Autodesk Inventor part; units mm, degrees
ref_plane "YZ Plane" through (0, 0, 0) normal (1, 0, 0) x (0, 1, 0)
ref_plane "XZ Plane" through (0, 0, 0) normal (0, 1, 0) x (-1, 0, 0)
ref_plane "XY Plane" through (0, 0, 0) normal (0, 0, 1) x (1, 0, 0)
sketch "Sketch1" plane through (0, 0, 0) normal (0, 1, 0) x (-1, 0, 0)
  line L0 (0, 0) -> (0, -152.4)
  line L1 (0, -152.4) -> (203.2, -152.4)
  line L2 (203.2, -152.4) -> (203.2, -31.75)
  line L3 (203.2, -31.75) -> (127, 0)
  line L4 (127, 0) -> (0, 0)
  dimension "d0" = 120.65
  dimension "d1" = 203.2
  dimension "d2" = 127
  dimension "d3" = 152.4
extrude "Extrusion1" add sketch "Sketch1" along normal blind 6.35
sketch "Sketch3" plane through (0, 6.35, 0) normal (0, 1, 0) x (1, 0, 0)
  line L0 (0, 0) -> (0, 152.4)
  line L1 (0, 152.4) -> (-203.2, 152.4)
  line L2 (-203.2, 152.4) -> (-203.2, 31.75)
  line L3 (-203.2, 31.75) -> (-127, 0)
  line L4 (-127, 0) -> (0, 0)
  line L5 (-19.05, 19.05) -> (-19.05, 133.35)
  line L6 (-19.05, 133.35) -> (-184.15, 133.35)
  line L7 (-184.15, 133.35) -> (-184.15, 50.8)
  line L8 (-19.05, 19.05) -> (-107.95, 19.05)
  line L9 (-107.95, 19.05) -> (-184.15, 50.8)
  circle A0 centre (-9.271, 15.875) radius 1.524
  circle A1 centre (-9.271, 136.525) radius 1.524
  circle A2 centre (-25.4, 143.129) radius 1.524
  circle A3 centre (-190.5, 143.129) radius 1.524
  circle A4 centre (-193.929, 47.625) radius 1.524
  circle A5 centre (-193.929, 136.525) radius 1.524
  circle A6 centre (-15.875, 9.271) radius 1.524
  circle A7 centre (-111.125, 9.271) radius 1.524
  dimension "d10" = 120.65
  dimension "d11" = 82.55
  dimension "d12" = 203.2
  dimension "d13" = 165.1
  dimension "d14" = 114.3
  dimension "d15" = 88.9
  dimension "d16" = 19.05
  dimension "d17" = 19.05
  dimension "d18" = 3.048
  dimension "d19" = 3.048
  dimension "d20" = 120.65
  dimension "d21" = 3.048
  dimension "d22" = 3.048
  dimension "d23" = 15.875
  dimension "d24" = 9.271
  dimension "d25" = 9.271
  dimension "d26" = 9.271
  dimension "d27" = 25.4
  dimension "d28" = 12.7
  dimension "d29" = 9.271
  dimension "d30" = 3.048
  dimension "d31" = 3.048
  dimension "d32" = 88.9
  dimension "d33" = 15.875
  dimension "d34" = 9.271
  dimension "d35" = 9.271
  dimension "d36" = 3.048
  dimension "d37" = 9.271
  dimension "d38" = 15.875
  dimension "d39" = 3.048
  dimension "d40" = 15.875
  dimension "d41" = 9.271
extrude "Extrusion2" cut sketch "Sketch3" against normal blind 6.35 contours L8 L9 L7 L6 L5 | A0 | A1 | A2 | A3 | A4 | A5 | A6 | A7
sketch "Sketch4" plane through (0, 6.35, 0) normal (0, 1, 0) x (1, 0, 0)
  circle A0 centre (-13.97, 44.45) radius 1.524
  circle A1 centre (-13.97, 107.95) radius 1.524
  circle A2 centre (-189.23, 92.075) radius 1.524
  line L0 (-107.95, 19.05) -> (-184.15, 50.8)
  line L1 (-184.15, 50.8) -> (-184.15, 133.35)
  line L2 (-19.05, 133.35) -> (-19.05, 19.05)
  point P0 (0, 0)
  dimension "d44" = 3.048
  dimension "d45" = 3.048
  dimension "d46" = 3.048
  dimension "d47" = 82.55
  dimension "d48" = 41.275
  dimension "d49" = 5.08
  dimension "d50" = 25.4
  dimension "d51" = 25.4
  dimension "d52" = 5.08
  dimension "d53" = 5.08
extrude "Extrusion3" cut sketch "Sketch4" against normal blind 6.35
properties part number "Panel"
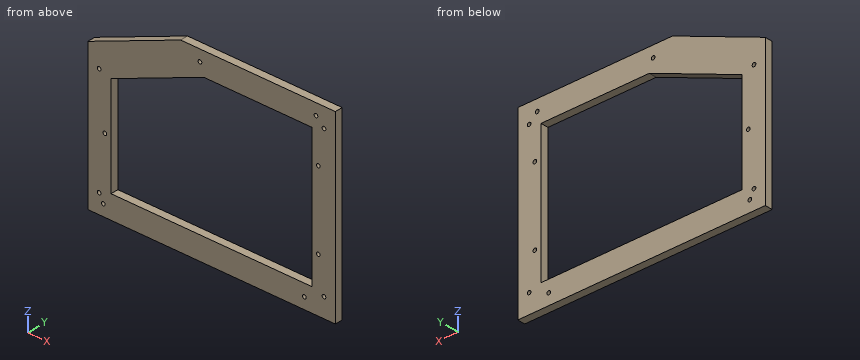
Design review of the part built by this model. Coordinates are the model's own, in mm. Give positions to 0.01 mm unless a question says otherwise; leave off trailing zeros. Write each loop counter-clockwise with the first axis right and the second up, starting at its lowest first coordinate (ties: lowest second). Pieces come first, ordered by that corner, then holes. Notation, with made-up numbers: (-36, 68.5) - (-11, 68.5) arc R26 ccw to (-11, 107.5) - close; hole circle Ø5 at (32.25, 64.25). An arc over 180 degrees is marked (long way). Return JSON: item names as keys, results as strings. Group by question number.
(1) We need section B-B, the plane x = -41. Give the boundary of the cut face in (y, z).
(2) We need section C-C, the plane y = 4. Give the number of separate pieces and of enclosed holes in the cut face, then the cut area to 3 significant figures.
(3) To check wall thickness, follow probe 1 along Z at (x, y) = (-13.97, 4.25); probe 2 along X at (y, z) = (1.5, -107.95); probe 3 along X at (y, z) = (4.25, -130). State the ranges of each line that lie inside material, in increasing order.
(4) We need section A-A, the plane z = -24. Give the boundary of the cut face in (x, y), then the cut area to 3 significant figures.
(5) Insertion check: pin 1 (3.5 mm diameter, centred on x = -189.23, z = -92.075, fed in from +Y). The pin has a flat end and moves straight along its axis. Give the tip position at first contact, or say it passes through.
Reported:
{
 "1": {"outline": "(0, -152.4) - (6.35, -152.4) - (6.35, -133.35) - (0, -133.35) - close; (0, -19.05) - (6.35, -19.05) - (6.35, 0) - (0, 0) - close"},
 "2": {"separate pieces": "1", "enclosed holes": "12", "area": "12,000 mm2"},
 "3": {"probe 1": "z = -152.4 to -109.47, -106.43 to -45.97, -42.93 to 0", "probe 2": "x = -203.2 to -184.15, -19.05 to -15.49, -12.45 to 0", "probe 3": "x = -203.2 to -184.15, -19.05 to 0"},
 "4": {"outline": "(-184.6, 0) - (-119.83, 0) - (-119.83, 6.35) - (-184.6, 6.35) - close; (-19.05, 0) - (0, 0) - (0, 6.35) - (-19.05, 6.35) - close", "area": "532 mm2"},
 "5": {"pin 1": "stops at y = 6.35"}
}
